For this review, take the finished solid that the model builds, in its own axes (mm). A direction names the side the tool comes from. Round coordinates to 2 decimals unless told otherwise and drop trailing zeros. Write each loop counter-clockwise with the first axis right and the second up, starting at its lowest first coordinate (ties: lowest second). Pieces come first, ordered by that corner, then holes. Notation, with made-up numbers: (48, 10.5) - (101, 10.5) arc R23 ccw to (101, 39.5) - close; hole circle Ø10 at (46, 26.25). An arc over 180 degrees is marked (long way). One line per item, written item: value. Start each with the question number.
Q1. Add section B-B on x = -15. Write out the cut boundary in (y, z).
Q2. Add section A-A on y = 25.5. Write out the cut boundary in (x, z), and give its area (3 significant figures).
Q3. For probe 1 along Y at (x, z) = (-7, 5.5); probe 2 along X at (y, z) = (16.5, 15.5); probe 3 along X at (y, z) = (16, 8.5), list the stretches that pass through material, from the lowest coordinate up.
Q4. Mouldability with a two-part tool opening along Y and no side actions: class faces 4 (the face through (-6, -27, 5)), 5 (the face through (-14, -50, 13)), 6 (the face through (-14.3, -0.7, 11.47)) as +Y half, -Y half, draft (parallel to the pull), parting line (faces both ways), or undercut.
Q5. Add section C-C on z = 4.5. Write out the cut boundary in (x, y), and give its area (3 significant figures).
Q6. Add section D-D on y = 38. Write out the cut boundary in (x, z), and give its area (3 significant figures).
Q7. Tool access review of faces 1 (the face through (-6, 28, 5)), 2 (the face through (-17, -28, 16)), 3 (the face through (-29, -1, 28)): name each direction out of +Z, -Z, +X, -X, +Y, -Y from which nothing blocks a thin tool from reaching the whole face with its end or side.
Q8. Clearance check with flat-ended pins moving along their axes: pin 1 Ø3 at (y, z) = (27.5, 15.5) entering from +X; pin 2 Ø3 at (y, z) = (25.5, 20) entering from +X; pin 3 Ø1.4 at (y, z) = (25, 4.5) entering from -X; pin 4 Ø8 at (x, z) = (-12.5, 22.5) entering from +Y. State where each tip first meets the part, or that it passes through.
Autodesk Inventor part; units mm, degrees
ref_plane "YZ Plane" through (0, 0, 0) normal (1, 0, 0) x (0, 1, 0)
ref_plane "XZ Plane" through (0, 0, 0) normal (0, 1, 0) x (-1, 0, 0)
ref_plane "XY Plane" through (0, 0, 0) normal (0, 0, 1) x (1, 0, 0)
sketch "Sketch1" plane through (0, 0, 0) normal (0, 1, 0) x (-1, 0, 0)
  line L0 (0, 0) -> (0, -2.8284)
  line L1 (0, -2.8284) -> (29, 26.1716)
  line L2 (29, 26.1716) -> (29, 29)
  line L3 (29, 29) -> (0, 0)
  dimension "d2" = 29
  dimension "d3" = 45
  dimension "d6" = 2
extrude "Extrusion1" add sketch "Sketch1" along normal mid plane 100
sketch "Sketch2" plane through (0, 0, 0) normal (0, 0, 1) x (1, 0, 0)
  line L0 (-17, 36) -> (-6, 36)
  line L1 (-6, 36) -> (-6, 19)
  line L2 (-6, 19) -> (-17, 19)
  line L3 (-17, 19) -> (-17, 36)
  line L4 (0, 50) -> (-29, 50)
  line L5 (0, -50) -> (0, 50)
  point P0 (0, 0)
  dimension "d7" = 14
  dimension "d8" = 17
  dimension "d9" = 11
  dimension "d11" = 6
extrude "Extrusion2" cut sketch "Sketch2" along normal up to next
mirror "Mirror1" about plane through (0, 0, 0) normal (0, 1, 0) of "Extrusion2"
sketch "Sketch3" plane through (0, -50, 0) normal (0.7071, 0, 0.7071) x (0.7071, 0, -0.7071)
  circle A0 centre (-30.5122, 5) radius 1.25
  circle A1 centre (-15.5122, 5) radius 1.25
  line L0 (-39.0122, 0) -> (-39.0122, 100)
  line L1 (-41.0122, 0) -> (-41.0122, 100)
  line L2 (0, 0) -> (-41.0122, 0)
  point P0 (0, 50)
  dimension "d15" = 5
  dimension "d16" = 2.5
  dimension "d17" = 15
  dimension "d18" = 2.5
  dimension "d19" = 5
  dimension "d20" = 10.5
extrude "Extrusion3" cut sketch "Sketch3" against normal up to next
mirror "Mirror2" about plane through (0, 0, 0) normal (0, 1, 0) of "Extrusion3"
properties part number "Front"
Result set:
1. outline: (-50, 12.17) - (-36, 12.17) - (-36, 15) - (-50, 15) - close; (-19, 12.17) - (19, 12.17) - (19, 15) - (-19, 15) - close; (36, 12.17) - (50, 12.17) - (50, 15) - (36, 15) - close
2. outline: (-29, 26.17) - (-17, 14.17) - (-17, 17) - (-29, 29) - close; (-6, 3.17) - (0, -2.83) - (0, 0) - (-6, 6) - close
2. area: 50.9 mm^2
3. probe 1: y = -50 to -36, -19 to 19, 36 to 50
3. probe 2: x = -18.33 to -15.5
3. probe 3: x = -11.33 to -8.5
4. face 4: undercut
4. face 5: -Y half
4. face 6: draft
5. outline: (-7.33, -50) - (-4.5, -50) - (-4.5, 50) - (-7.33, 50) - (-7.33, 36) - (-6, 36) - (-6, 19) - (-7.33, 19) - (-7.33, -19) - (-6, -19) - (-6, -36) - (-7.33, -36) - close
5. area: 238 mm^2
6. outline: (-29, 26.17) - (0, -2.83) - (0, 0) - (-29, 29) - close
6. area: 82.0 mm^2
7. face 1: +Z, -Z, -X
7. face 2: +Z, -Z, +X
7. face 3: +Z, -Z, -X, +Y, -Y
8. pin 1: stops at x = -17
8. pin 2: stops at x = -18.5
8. pin 3: stops at x = -6
8. pin 4: passes through
